Read the model definition and answer for the solid it produces. Units are mm, in the model's axes. Face numbers are marked on the shaded views. Give positions to 0.01 mm unless a question says otherwise; leave off trailing zeros. Loops run counter-clockwise (first coordinate to the right, second up) from the corner with the lowest first, then second, coordinate; pieces in that order, holes last. Notation, with made-up numbers: M 67,37 L 90,37 A27 ccw 90,70 Z; hole C 31,50 d1. An arc over 180 degrees is marked long. Return JSON: item names as keys, results as strings. Group by question number.
```python
from build123d import *

# Parameters (mm, degrees)
EXTRUDE_1_DEPTH      = 3
SKETCH_2_W           = 12
SKETCH_2_H           = 12.5
EXTRUDE_2_DEPTH      = 4
EXTRUDE_3_DEPTH      = 3
SKETCH_4_R           = 3.25
CUT_EXTRUDE_1_DEPTH  = 13.5
EXTRUDE_4_DEPTH      = 2
EXTRUDE_4_DEPTH_BACK = 2
SKETCH_6_R           = 3.5
EXTRUDE_5_DEPTH      = 20


with BuildPart() as part:
    # Эскиз1 → Бобышка-Вытянуть1 (new body)
    with BuildSketch(Plane(origin=(0, 0, 0), x_dir=(1, 0, 0), z_dir=(0, 1, 0))):
        with BuildLine():
            Line((-7.38128575, -1.329142833), (-6, -9))
            Line((-6, -9), (6, -9))
            Line((6, -9), (7.38128575, -1.329142833))
            ThreePointArc((7.38128575, -1.329142833), (0, 7.5), (-7.38128575, -1.329142833))
        make_face()
    extrude(amount=EXTRUDE_1_DEPTH)

    # Эскиз2 → Бобышка-Вытянуть2 (add)
    with BuildSketch(Plane.XY.offset(9)):
        with Locations((0, 6.25)):
            Rectangle(SKETCH_2_W, SKETCH_2_H)
    extrude(amount=EXTRUDE_2_DEPTH)

    # Эскиз3 → Бобышка-Вытянуть3 (add)
    with BuildSketch(Plane(origin=(0, 12.5, 0), x_dir=(1, 0, 0), z_dir=(0, 1, 0))):
        with BuildLine():
            Line((-7.38128575, -1.329142833), (-6, -9))
            Line((-6, -9), (6, -9))
            Line((6, -9), (7.38128575, -1.329142833))
            ThreePointArc((7.38128575, -1.329142833), (0, 7.5), (-7.38128575, -1.329142833))
        make_face()
    extrude(amount=-EXTRUDE_3_DEPTH)

    # Эскиз4 → Вырез-Вытянуть1 (cut, through all)
    with BuildSketch(Plane(origin=(0, 12.5, 0), x_dir=(1, 0, 0), z_dir=(0, 1, 0))):
        Circle(SKETCH_4_R)
    extrude(amount=-CUT_EXTRUDE_1_DEPTH, mode=Mode.SUBTRACT)

    # Эскиз5 → Бобышка-Вытянуть4 (add, two sides)
    with BuildSketch(Plane(origin=(0, 6.25, 0), x_dir=(1, 0, 0), z_dir=(0, 1, 0))) as extrude_4_sk:
        with BuildLine():
            Line((-6, -13), (6, -13))
            Line((6, -13), (6, -134.006168685))
            Line((6, -134.006168685), (3.418398609, -145.751366054))
            ThreePointArc((3.418398609, -145.751366054), (0, -148.5), (-3.418398609, -145.751366054))
            Line((-3.418398609, -145.751366054), (-6, -134.006168685))
            Line((-6, -134.006168685), (-6, -13))
        make_face()
        with BuildLine():
            Line((3.5, -38), (3.5, -48))
            ThreePointArc((3.5, -48), (0, -51.5), (-3.5, -48))
            Line((-3.5, -48), (-3.5, -38))
            ThreePointArc((-3.5, -38), (0, -34.5), (3.5, -38))
        make_face(mode=Mode.SUBTRACT)
    extrude(amount=EXTRUDE_4_DEPTH)
    extrude(extrude_4_sk.sketch, amount=-EXTRUDE_4_DEPTH_BACK)

    # Эскиз6 → Бобышка-Вытянуть5 (add)
    with BuildSketch(Plane(origin=(0, 8.25, 0), x_dir=(1, 0, 0), z_dir=(0, 1, 0))):
        with Locations((0, -145)):
            Circle(SKETCH_6_R)
    extrude(amount=-EXTRUDE_5_DEPTH)


solid = part.part
```
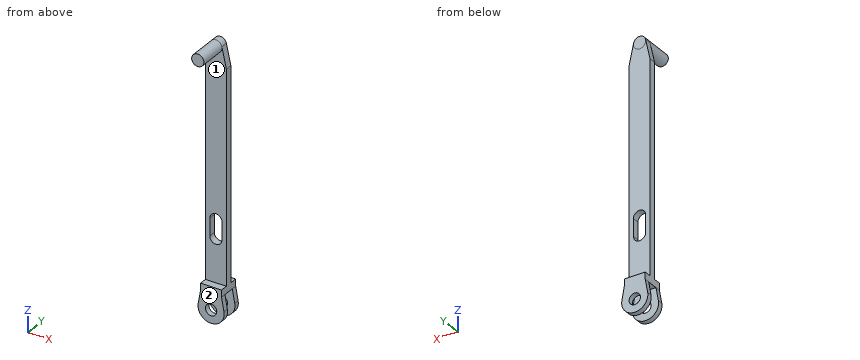
1. Flat-ended cylindrical pins translate along their axes: P1, Ø3.5, axis at x = -1, z = 55.5, coming from the +Y side; P2, Ø6, axis at y = 6.5, z = 72, coming from the -X side; P3, Ø14, axis at y = 9, z = 52, coming from the +X side. Find the tip coordinate at first contact, or state that the pin passes through.
2. Straight lines are drawn through the part: line 1 along Z through (x, y) = (0, 1.6); line 2 along Z through (x, y) = (0, 10.75); line 3 along X through (y, z) = (10.6, 0). For each, find the intervals that lie inside material, in ascending order.
3. The mould has two halves that part along Z. Classify the marked faces 1 and 2: +Z half, -Z half, draft (parallel to the pull), parting line (faces both ways), or undercut.
4. Find section A-A (x = 0). Write down the section's boundary in (y, z), and give its area (3 significant figures).
5. Find section C-C (y = -5). Write down the section's boundary in (x, z).
6. Find section D-D (z = 30). Write down the section's boundary in (x, y).
7. Find section B-B (z = 0). Write down the section's boundary in (x, y), and give its area (3 significant figures).
Result:
{
 "1": {"P1": "stops at y = 8.25", "P2": "stops at x = -6", "P3": "stops at x = 6"},
 "2": {"line 1": "z = -7.5 to -3.25, 3.25 to 13, 141.5 to 148.5", "line 2": "z = -7.5 to -3.25, 3.25 to 13", "line 3": "x = -7.5 to -3.25, 3.25 to 7.5"},
 "3": {"face 1": "undercut", "face 2": "draft"},
 "4": {"outline": "M -11.75,141.5 L 4.25,141.5 L 4.25,51.5 L 8.25,51.5 L 8.25,148.5 L -11.75,148.5 Z; M 0,-7.5 L 3,-7.5 L 3,-3.25 L 0,-3.25 Z; M 0,3.25 L 3,3.25 L 3,9 L 9.5,9 L 9.5,3.25 L 12.5,3.25 L 12.5,13 L 8.25,13 L 8.25,34.5 L 4.25,34.5 L 4.25,13 L 0,13 Z; M 9.5,-7.5 L 12.5,-7.5 L 12.5,-3.25 L 9.5,-3.25 Z", "area": "696 mm2"},
 "5": {"outline": "C 0,145 d7"},
 "6": {"outline": "M -6,4.25 L 6,4.25 L 6,8.25 L -6,8.25 Z"},
 "7": {"outline": "M -7.5,0 L -3.25,0 L -3.25,3 L -7.5,3 Z; M -7.5,9.5 L -3.25,9.5 L -3.25,12.5 L -7.5,12.5 Z; M 3.25,0 L 7.5,0 L 7.5,3 L 3.25,3 Z; M 3.25,9.5 L 7.5,9.5 L 7.5,12.5 L 3.25,12.5 Z", "area": "51.0 mm2"}
}
